from build123d import *

# Parameters (mm, degrees)
SKETCH1_R            = 95
SKETCH1_R_2          = 70
BOSS_EXTRUDE1_DEPTH  = 44
CUT_EXTRUDE3_DEPTH   = 15
CIRPATTERN2_COUNT    = 6
M3_CLEARANCE_HOLE1_D = 3.2
M3_CLEARANCE_HOLE2_D = 3.2


with BuildPart() as part:
    # Sketch1 → Boss-Extrude1 (new body)
    with BuildSketch(Plane(origin=(0, 0, 0), x_dir=(1, 0, 0), z_dir=(0, 1, 0))):
        with Locations(Location((0, 0, 0), (0, 0, 270))):
            Circle(SKETCH1_R)
        with Locations(Location((0, 0, 0), (0, 0, 270))):
            Circle(SKETCH1_R_2, mode=Mode.SUBTRACT)
    extrude(amount=BOSS_EXTRUDE1_DEPTH)

    # Sketch7 → Cut-Extrude3 (cut, symmetric)
    with BuildSketch(Plane(origin=(0, 0, 0), x_dir=(0, -1, 0), z_dir=(-0.500000000000001, 0, 0.866025403784438))):
        Polygon((-44, 83), (-34, 83), (-29, 78), (-34, 73), (-44, 73), align=None)
        Polygon((-10, 83), (0, 83), (0, 73), (-10, 73), (-15, 78), align=None)
    cut_extrude3 = extrude(amount=CUT_EXTRUDE3_DEPTH, both=True, mode=Mode.SUBTRACT)

    # CirPattern2: Cut-Extrude3 ×6 about axis
    cirpattern2_axis = Axis((0, 0, 0), (0, 1, 0))
    for i in range(1, CIRPATTERN2_COUNT):
        add(cut_extrude3.rotate(cirpattern2_axis, i * 360 / CIRPATTERN2_COUNT), mode=Mode.SUBTRACT)

    # M3 Clearance Hole1 (through all)
    with Locations(Plane(origin=(0, 44, 0), x_dir=(1, 0, 0), z_dir=(0, 1, 0))):
        with Locations((62.549981495, -47.660254038), (72.549981495, -30.339745962), (-10, -78), (10, -78), (-72.549981495, -30.339745962), (-62.549981495, -47.660254038), (-62.549981495, 47.660254038), (-72.549981495, 30.339745962), (10, 78), (-10, 78), (72.549981495, 30.339745962), (62.549981495, 47.660254038), (0, 0)):
            Hole(M3_CLEARANCE_HOLE1_D / 2)

    # M3 Clearance Hole2 (through all)
    with Locations(Plane(origin=(0, 44, 0), x_dir=(1, 0, 0), z_dir=(0, 1, 0))):
        with Locations((0, 90), (23.293714059, 86.933324366), (45, 77.942286341), (63.639610307, 63.639610307), (77.942286341, 45), (86.933324366, 23.293714059), (90, 0), (86.933324366, -23.293714059), (77.942286341, -45), (63.639610307, -63.639610307), (45, -77.942286341), (23.293714059, -86.933324366), (0, -90), (-23.293714059, -86.933324366), (-45, -77.942286341), (-63.639610307, -63.639610307), (-77.942286341, -45), (-86.933324366, -23.293714059), (-90, 0), (-86.933324366, 23.293714059), (-77.942286341, 45), (-63.639610307, 63.639610307), (-45, 77.942286341), (-23.293714059, 86.933324366), (0, 0)):
            Hole(M3_CLEARANCE_HOLE2_D / 2)


solid = part.part
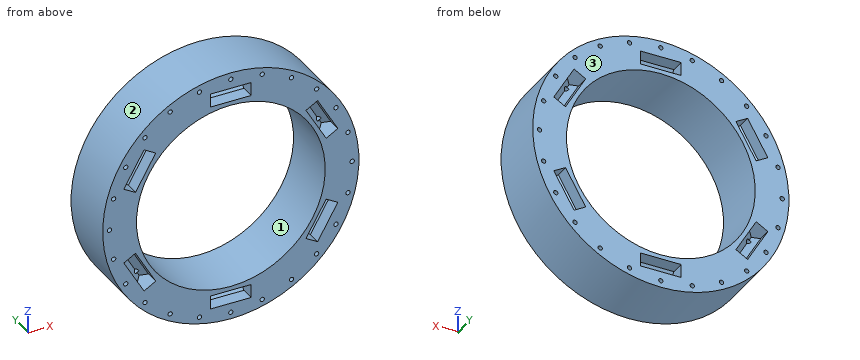
Work out the finished part from the listing and answer in its coordinate system (mm). Face numbers are marked on the shaded views. Give positions to 0.01 mm unless a question says otherwise; leave off trailing zeros. Order: outer loops, then holes, each group sorted by start corner. A loop starts at its lowest first (then second) coordinate and runs counter-clockwise, first axis right, second up. Notation, with made-up numbers: M -11.75,23.25 L 41.25,23.25 A14 ccw 41.25,50.25 Z; hole C 21,17 d7. An arc over 180 degrees is marked long. Return JSON: item names as keys, results as strings.
Q1. Find section B-B, the plane x = -19. Write down the section's boundary in (y, z).
Answer below:
{"outline": "M 0,-93.08 L 44,-93.08 L 44,-67.37 L 0,-67.37 Z; M 0,67.37 L 44,67.37 L 44,93.08 L 0,93.08 Z"}
Q2. Each of these flat-tipped pins is pushed along its axis until it touches: pin 1 (4 mm diameter, centred on x = 73, y = 21.5, fed in from +Z); pin 2 (2 mm diameter, centred on y = 32.5, z = 26, fed in from -X); pin 3 (8 mm diameter, centred on x = 6, y = 39, fed in from -Z). Where does it stop, or does it pass through?
Answer below:
{"pin 1": "stops at z = 63.12", "pin 2": "stops at x = -91.65", "pin 3": "stops at z = -94.98"}
Q3. Find section C-C, the plane y = 40. State how many separate pieces and enclosed holes the cut face has, and give its area (3 significant figures).
Answer below:
{"separate pieces": "1", "enclosed holes": "31", "area": "11,000 mm^2"}
Q4. The mould has two halves that part along Z. Classify the marked faces 1, 2 and 3: pulls with the +Z half, pulls with the -Z half, needs draft (parallel to the pull), parting line crosses it, or undercut.
Answer below:
{"face 1": "undercut", "face 2": "parting line crosses it", "face 3": "needs draft"}
Q5. Find section A-A, the plane z = 19. Write down the section's boundary in (x, y), and give its area (3 significant figures).
Answer below:
{"outline": "M -93.08,0 L -67.37,0 L -67.37,44 L -93.08,44 Z; M 67.37,0 L 93.08,0 L 93.08,44 L 67.37,44 Z", "area": "2,260 mm^2"}
Q6. Find the intervals of material crossed by line 1 along Z through (x, y) = (-10, 20.5); line 2 along X through (y, z) = (11.5, -78.5); line 3 along X through (y, z) = (32, -45), in increasing order. Write a range as [from, to].
Answer below:
{"line 1": "z = [-94.47, -79.6], [-76.4, -69.28], [69.28, 76.4], [79.6, 94.47]", "line 2": "x = [-53.5, -46.5], [-43.5, -15], [15, 43.5], [46.5, 53.5]", "line 3": "x = [-83.67, -79.54], [-76.34, -67.55], [-60.62, -53.62], [53.62, 60.62], [67.55, 76.34], [79.54, 83.67]"}
